CAD build for the part. Positions are in the model's coordinates, mm. A direction names the side the tool comes from. Give positions to 0.01 mm unless a question says otherwise; leave off trailing zeros. Loops run counter-clockwise (first coordinate to the right, second up) from the corner with the lowest first, then second, coordinate; pieces in that order, holes last.
```python
from build123d import *

# Parameters (mm, degrees)
BOSS_EXTRUDE1_DEPTH = 3
SKETCH2_R           = 1.5
CUT_EXTRUDE1_DEPTH  = 3
SKETCH3_W           = 20
SKETCH3_H           = 3
SKETCH3_W_2         = 14
CUT_EXTRUDE2_DEPTH  = 3
SKETCH4_W           = 14
SKETCH4_H           = 8
CUT_EXTRUDE3_DEPTH  = 3
SKETCH5_R           = 1.5
CUT_EXTRUDE4_DEPTH  = 3


with BuildPart() as part:
    # Sketch1 → Boss-Extrude1 (new body)
    with BuildSketch(Plane.XY):
        with BuildLine():
            Line((10.270588235, 0.331568073), (10.270588235, -27.668431927))
            ThreePointArc((10.270588235, -27.668431927), (9.684801798, -29.08264549), (8.270588235, -29.668431927))
            Line((8.270588235, -29.668431927), (-15.729411765, -29.668431927))
            ThreePointArc((-15.729411765, -29.668431927), (-19.09389159, -28.274818754), (-20.487504763, -24.910338929))
            Line((-20.487504763, -24.910338929), (-20.487504763, -14.033468446))
            ThreePointArc((-20.487504763, -14.033468446), (-20.916042168, -12.389775022), (-22.453909691, -11.668431927))
            Line((-22.453909691, -11.668431927), (-29.729411765, -11.668431927))
            ThreePointArc((-29.729411765, -11.668431927), (-36.800479577, -8.739499739), (-39.729411765, -1.668431927))
            ThreePointArc((-39.729411765, -1.668431927), (-36.800479577, 5.402635884), (-29.729411765, 8.331568073))
            ThreePointArc((-29.729411765, 8.331568073), (-25.969894889, 7.597960729), (-22.761979852, 5.504774645))
            ThreePointArc((-22.761979852, 5.504774645), (-20.403371026, 3.939172769), (-17.6384187, 3.331568073))
            Line((-17.6384187, 3.331568073), (7.270588235, 3.331568073))
            ThreePointArc((7.270588235, 3.331568073), (9.391908579, 2.452888416), (10.270588235, 0.331568073))
        make_face()
    extrude(amount=BOSS_EXTRUDE1_DEPTH)

    # Sketch2 → Cut-Extrude1 (cut)
    with BuildSketch(Plane.XY.offset(3)):
        with Locations((-29.729411765, -1.668431927)):
            Circle(SKETCH2_R)
    extrude(amount=-CUT_EXTRUDE1_DEPTH, mode=Mode.SUBTRACT)

    # Sketch3 → Cut-Extrude2 (cut)
    with BuildSketch(Plane.XY.offset(3)):
        with Locations((-4.729411765, -10.168431927)):
            Rectangle(SKETCH3_W, SKETCH3_H)
        with Locations((3.270588235, -17.468431927)):
            Rectangle(SKETCH3_W_2, SKETCH3_H)
        with Locations((3.270588235, -23.768431927)):
            Rectangle(SKETCH3_W_2, SKETCH3_H)
    extrude(amount=-CUT_EXTRUDE2_DEPTH, mode=Mode.SUBTRACT)

    # Sketch4 → Cut-Extrude3 (cut)
    with BuildSketch(Plane.XY.offset(3)):
        with Locations((-3.729411765, -4.668431927)):
            Rectangle(SKETCH4_W, SKETCH4_H)
    extrude(amount=-CUT_EXTRUDE3_DEPTH, mode=Mode.SUBTRACT)

    # Sketch5 → Cut-Extrude4 (cut)
    with BuildSketch(Plane.XY.offset(3)):
        with Locations((-14.229411765, -2.968431927)):
            Circle(SKETCH5_R)
    extrude(amount=-CUT_EXTRUDE4_DEPTH, mode=Mode.SUBTRACT)


solid = part.part
```
1. Saw through at C-C, the plane x = 2. List the corners of the cut face in (y, z), and give its area (3 significant figures).
Responses:
outline: (-29.67, 0) - (-25.27, 0) - (-25.27, 3) - (-29.67, 3) - close; (-22.27, 0) - (-18.97, 0) - (-18.97, 3) - (-22.27, 3) - close; (-15.97, 0) - (-11.67, 0) - (-11.67, 3) - (-15.97, 3) - close; (-0.67, 0) - (3.33, 0) - (3.33, 3) - (-0.67, 3) - close
area: 48.0 mm2
2. Saw through at D-D, the plane z = 1.3. Count the separate pieces of the cut face and the enclosed holes in it, and give its area (3 significant figures).
Responses:
separate pieces: 1
enclosed holes: 3
area: 1,070 mm2
3. Saw through at B-B, the plane y = -11. List the corners of the cut face in (x, z), and give its area (3 significant figures).
Responses:
outline: (-33.32, 0) - (-14.73, 0) - (-14.73, 3) - (-33.32, 3) - close; (5.27, 0) - (10.27, 0) - (10.27, 3) - (5.27, 3) - close
area: 70.8 mm2
4. Saw through at A-A, the plane x = -11.5. List the corners of the cut face in (y, z), and give its area (3 significant figures).
Responses:
outline: (-29.67, 0) - (-11.67, 0) - (-11.67, 3) - (-29.67, 3) - close; (-8.67, 0) - (3.33, 0) - (3.33, 3) - (-8.67, 3) - close
area: 90.0 mm2
5. Pull direction X, two halves, no side cores. Call faces 1 (the face through (3, -25.268, 2)), 2 (the face through (-3.729, -24, 2)), 3 (the face through (-5, -11.668, 2)), 4 (the face through (-28.3, -1.22, 1.52)): released by +X, released by -X, zero draft, split by the parting line, or undercut.
Responses:
face 1: zero draft
face 2: released by +X
face 3: undercut
face 4: undercut
6. Tool access for faces 5 (the face through (-14.729, -10, 2)), 6 (the face through (-20.488, -20, 1)), 7 (the face through (3, -15.968, 2)): list every direction of +Z, -Z, +X, -X, +Y, -Y with a clear straight run to the whole face (end or side of a thin tool).
Responses:
face 5: +Z, -Z
face 6: +Z, -Z, -X, -Y
face 7: +Z, -Z, +X
7. Drop flat-ended pins along their axis: pin 1 (0.9 mm diameter, centred on x = 3.5, z = 1.5, fed in from +Y); pin 2 (0.9 mm diameter, centred on y = -18, z = 2, fed in from +X); pin 3 (0.9 mm diameter, centred on y = -3, z = 1.5, fed in from -X). Give the stop position or say it passes through.
Responses:
pin 1: stops at y = 3.33
pin 2: stops at x = -3.73
pin 3: stops at x = -39.69
8. Probe line 1 along Y through (x, z) = (-3, 0.8); line 2 along Y through (x, z) = (-7, 2.4); line 3 along X through (y, z) = (-1, 2.4). List the from-to ranges inside material, lowest first.
Responses:
line 1: y = -29.67 to -25.27, -22.27 to -18.97, -15.97 to -11.67, -0.67 to 3.33
line 2: y = -29.67 to -11.67, -0.67 to 3.33
line 3: x = -39.71 to -31.07, -28.39 to -10.73, 3.27 to 10.27
